from build123d import *

# Parameters (mm, degrees)
BOSS_EXTRUDE1_DEPTH = 1009.525
SKETCH3_W           = 1919.05
SKETCH3_H           = 40.475
BOSS_EXTRUDE2_DEPTH = 19.05
FILLET1_R           = 55
BOSS_EXTRUDE4_START = -50
SKETCH4_W           = 2000
SKETCH4_H           = 40.475
BOSS_EXTRUDE4_DEPTH = 69.05
BOSS_EXTRUDE6_START = 19.05
SKETCH6_W           = 2000
SKETCH6_H           = 25
BOSS_EXTRUDE6_DEPTH = 32
CUT_EXTRUDE5_START  = 1050
SKETCH5_R           = 10.16
CUT_EXTRUDE5_DEPTH  = 25
SKETCH7_W           = 10
SKETCH7_H           = 101.05
CUT_EXTRUDE6_DEPTH  = 1451.89837773


with BuildPart() as part:
    # Sketch2 → Boss-Extrude1 (new body)
    with BuildSketch(Plane.XY):
        Polygon((-959.525, 0), (959.525, 0), (959.525, 19.05), (1000, 19.05), (1000, -50), (-1000, -50), (-1000, 19.05), (-959.525, 19.05), align=None)
    extrude(amount=BOSS_EXTRUDE1_DEPTH)

    # Sketch3 → Boss-Extrude2 (add)
    with BuildSketch(Plane(origin=(0, 0, 0), x_dir=(1, 0, 0), z_dir=(0, 1, 0))):
        with Locations((0, -20.2375)):
            Rectangle(SKETCH3_W, SKETCH3_H)
    extrude(amount=BOSS_EXTRUDE2_DEPTH)

    # Fillet1
    fillet1_edges = [part.edges().sort_by_distance(p)[0] for p in [
        (959.525, 9.525, 40.475),
        (-959.525, 9.525, 40.475),
    ]]
    fillet(fillet1_edges, radius=FILLET1_R)

    # Sketch4 → Boss-Extrude4 (add)
    with BuildSketch(Plane(origin=(0, 0, 0), x_dir=(1, 0, 0), z_dir=(0, 1, 0)).offset(BOSS_EXTRUDE4_START)):
        with Locations((0, -1029.7625)):
            Rectangle(SKETCH4_W, SKETCH4_H)
    extrude(amount=BOSS_EXTRUDE4_DEPTH)

    # Sketch6 → Boss-Extrude6 (add)
    with BuildSketch(Plane(origin=(0, 0, 0), x_dir=(1, 0, 0), z_dir=(0, 1, 0)).offset(BOSS_EXTRUDE6_START)):
        with Locations((0, -12.5)):
            Rectangle(SKETCH6_W, SKETCH6_H)
        with Locations((0, -1037.5)):
            Rectangle(SKETCH6_W, SKETCH6_H)
    extrude(amount=BOSS_EXTRUDE6_DEPTH)

    # Sketch5 → Cut-Extrude5 (cut)
    with BuildSketch(Plane.XY.offset(CUT_EXTRUDE5_START)):
        with Locations(Location((-950, 9.525, 0), (0, 0, 69.635865194))):
            Circle(SKETCH5_R)
        with Locations(Location((950, 9.525, 0), (0, 0, 69.635865194))):
            Circle(SKETCH5_R)
    extrude(amount=-CUT_EXTRUDE5_DEPTH, mode=Mode.SUBTRACT)

    # Sketch7 → Cut-Extrude6 (cut, through all)
    with BuildSketch(Plane.XY):
        with Locations((-995, 0.525)):
            Rectangle(SKETCH7_W, SKETCH7_H)
        with Locations((995, 0.525)):
            Rectangle(SKETCH7_W, SKETCH7_H)
    extrude(amount=CUT_EXTRUDE6_DEPTH, mode=Mode.SUBTRACT)


solid = part.part
Can you work these out from the model? Positions are in its coordinate system, mm. A direction names the side the tool comes from. Give positions to 0.01 mm unless a question says otherwise; leave off trailing zeros. Write each loop counter-clockwise with the first axis right and the second up, starting at its lowest first coordinate (ties: lowest second). Pieces come first, ordered by that corner, then holes. Notation, with made-up numbers: (12, -40) -> (28, -40) arc R21 ccw to (28, -7) -> close; hole circle Ø7 at (38, 25). An arc over 180 degrees is marked (long way). Answer as a JSON object with one key per item and string values. Group by question number.
Item 1: For faces 1 (the face through (942.986, 9.658, 56.159)), 2 (the face through (-14, 0, 0)), which set-ups out of +Z, -Z, +X, -X, +Y, -Y let a thin tool reach every point of the face, with its end or its side?
Item 2: We'd pull the mould along X, two halves only. Please class faces 3 (the face through (-13, 0, 518)), 4 (the face through (-14, -50, 518)), 5 (the face through (-942.986, 9.658, 56.159)), 6 (the face through (-990, -23, 518)): +X half, -X half, draft (parallel to the pull), parting line (faces both ways), or undercut.
Item 3: Suppose I cut it at B-B (z = 927.5). Please give me the cut outline in (x, y) (3 decimals), plus the area to 3 significant figures.
Item 4: Suppose I cut it at A-A (x = 752). Please give me the cut outline in (y, z) (3 decimals).
Item 5: Please list where these lines run through material, in increasing order: line 1 (Z direction, x = 31.5, y = 10.5) (3 decimals); line 2 (X direction, y = 17.5, z = 252) (3 decimals); line 3 (Y direction, x = -950, z = 1041.75) (3 decimals). Write a range as [from, to].
Item 6: I'm going to push flat-ended pins straight in: P1, Ø5.5, axis at x = 12, y = 8, coming from the -Z side; P2, Ø1.5, axis at x = 638.5, z = 150.5, coming from the +Y side; P3, Ø18.5, axis at x = -950, y = 9.525, coming from the +Z side. Where does each tip first touch, or does it pass through?
Findings:
{
 "1": {"face 1": "+Y", "face 2": "-Z, +X, -X, +Y, -Y"},
 "2": {"face 3": "undercut", "face 4": "draft", "face 5": "undercut", "face 6": "-X half"},
 "3": {"outline": "(-990, -50) -> (990, -50) -> (990, 19.05) -> (959.525, 19.05) -> (959.525, 0) -> (-959.525, 0) -> (-959.525, 19.05) -> (-990, 19.05) -> close", "area": "100,000 mm²"},
 "4": {"outline": "(-50, 0) -> (51.05, 0) -> (51.05, 25) -> (19.05, 25) -> (19.05, 40.475) -> (0, 40.475) -> (0, 1009.525) -> (19.05, 1009.525) -> (19.05, 1025) -> (51.05, 1025) -> (51.05, 1050) -> (-50, 1050) -> close"},
 "5": {"line 1": "z = [0, 40.475], [1009.525, 1050]", "line 2": "x = [-990, -959.525], [959.525, 990]", "line 3": "y = [-50, -0.635], [19.685, 51.05]"},
 "6": {"P1": "stops at z = 0", "P2": "stops at y = 0", "P3": "stops at z = 1025"}
}
